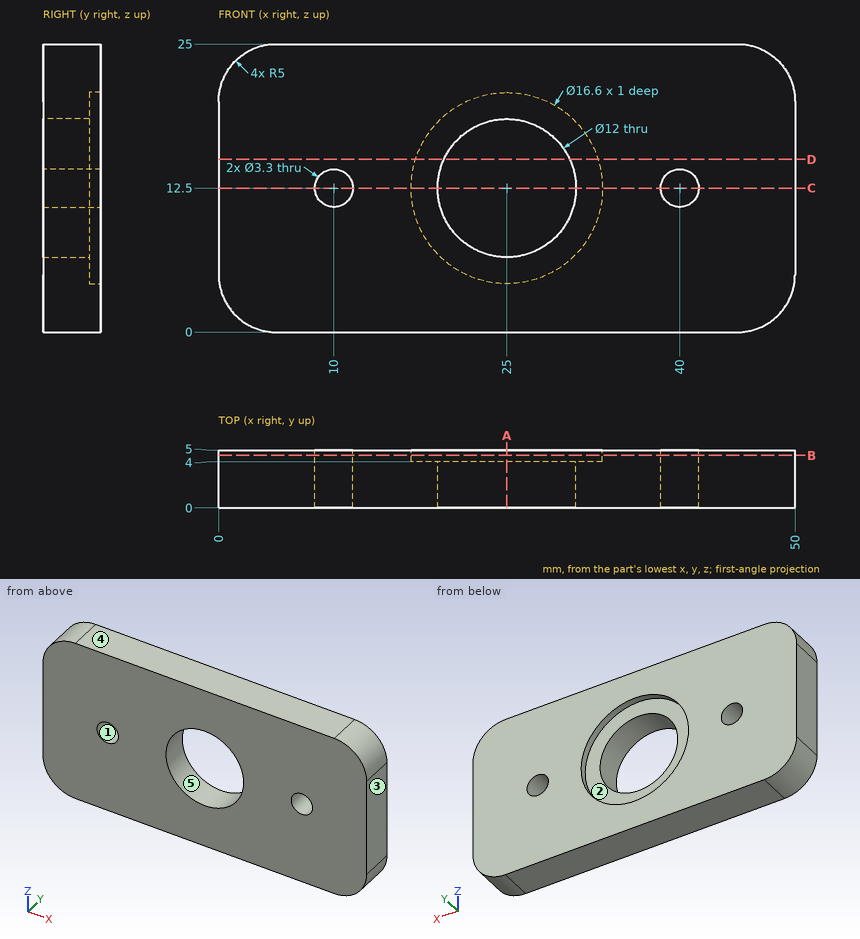
Could you check a few things on this drawing? It's one solid part, dimensions in mm from its lowest x, y, z. A direction names the side the tool comes from. Coordinates: 2 decimals unless noted, no trailing zeros. Write each loop counter-clockwise with the first axis right and the second up, starting at its lowest first coordinate (ties: lowest second). Pieces come first, ordered by that corner, then holes. Notation, with made-up numbers: (-11, 76) - (12, 76) arc R29 cw to (12, 99) - close; hole circle Ø7 at (41, 87). An arc over 180 degrees is marked (long way). Write item = value, one per line.
1) Suppose I cut it at D-D on z = 15. Please give me the cut outline in (x, y).
Result set:
outline = (0, 0) - (19.55, 0) - (19.55, 4) - (17.09, 4) - (17.09, 5) - (0, 5) - close; (30.45, 0) - (50, 0) - (50, 5) - (32.91, 5) - (32.91, 4) - (30.45, 4) - close
2) Suppose I cut it at C-C on z = 12.5. Please give me the cut outline in (x, y).
Result set:
outline = (0, 0) - (8.35, 0) - (8.35, 5) - (0, 5) - close; (11.65, 0) - (19, 0) - (19, 4) - (16.7, 4) - (16.7, 5) - (11.65, 5) - close; (31, 0) - (38.35, 0) - (38.35, 5) - (33.3, 5) - (33.3, 4) - (31, 4) - close; (41.65, 0) - (50, 0) - (50, 5) - (41.65, 5) - close
3) For the marked faces 1 and 2, which set-ups out of +Z, -Z, +X, -X, +Y, -Y let a thin tool reach every point of the face, with its end or its side?
Result set:
face_1 = +Y, -Y
face_2 = +Y
4) Suppose I cut it at A-A on x = 25. Please give me the cut outline in (y, z).
Result set:
outline = (0, 0) - (5, 0) - (5, 4.2) - (4, 4.2) - (4, 6.5) - (0, 6.5) - close; (0, 18.5) - (4, 18.5) - (4, 20.8) - (5, 20.8) - (5, 25) - (0, 25) - close
5) Will this pin go through, and if not, where does the flat tip stop? pin 1 Ø2 at (x, z) = (33, 14) entering from -Y.
Result set:
pin_1 = 0
6) We'd pull the mould along X, two halves only. Please class the marked faces 3, 4 and 5: +X half, -X half, draft (parallel to the pull), parting line (faces both ways), or undercut.
Result set:
face_3 = +X half
face_4 = draft
face_5 = undercut
7) Suppose I cut it at B-B on y = 4.55. Please give me the cut outline in (x, z), plus the area to 3 significant figures.
Result set:
outline = (0, 5) arc R5 ccw to (5, 0) - (45, 0) arc R5 ccw to (50, 5) - (50, 20) arc R5 ccw to (45, 25) - (5, 25) arc R5 ccw to (0, 20) - close; hole circle Ø3.3 at (10, 12.5); hole circle Ø16.6 at (25, 12.5); hole circle Ø3.3 at (40, 12.5)
area = 995 mm2
8) Please list where these lines run through material, in increasing order: line 1 (X direction, y = 1.1, z = 12.5); line 2 (X direction, y = 4.4, z = 12.5); line 3 (Z direction, x = 24, y = 2.8). Write a range as [from, to].
Result set:
line_1 = [0, 8.35], [11.65, 19], [31, 38.35], [41.65, 50]
line_2 = [0, 8.35], [11.65, 16.7], [33.3, 38.35], [41.65, 50]
line_3 = [0, 6.58], [18.42, 25]
